from build123d import *

# Parameters (mm, degrees)
BOSS_EXTRUDE1_DEPTH          = 2
SKETCH2_W                    = 2
SKETCH2_H                    = 25
CUT_EXTRUDE_THIN1_DEPTH      = 1
CUT_EXTRUDE_THIN1_DEPTH_BACK = 3


with BuildPart() as part:
    # Sketch1 → Boss-Extrude1 (new body)
    with BuildSketch(Plane(origin=(0, 0, 0), x_dir=(1, 0, 0), z_dir=(0, 1, 0))):
        Polygon((-20.207259422, -35), (20.207259422, -35), (40.414518843, 0), (20.207259422, 35), (-20.207259422, 35), (-40.414518843, 0), align=None)
    extrude(amount=BOSS_EXTRUDE1_DEPTH)

    # Sketch2 → Cut-Extrude-Thin1 (cut, two sides)
    with BuildSketch(Plane(origin=(0, 2, 0), x_dir=(1, 0, 0), z_dir=(0, 1, 0))) as cut_extrude_thin1_sk:
        with Locations((0, 12.5)):
            Rectangle(SKETCH2_W, SKETCH2_H)
    extrude(amount=CUT_EXTRUDE_THIN1_DEPTH, mode=Mode.SUBTRACT)
    extrude(cut_extrude_thin1_sk.sketch, amount=-CUT_EXTRUDE_THIN1_DEPTH_BACK, mode=Mode.SUBTRACT)


solid = part.part
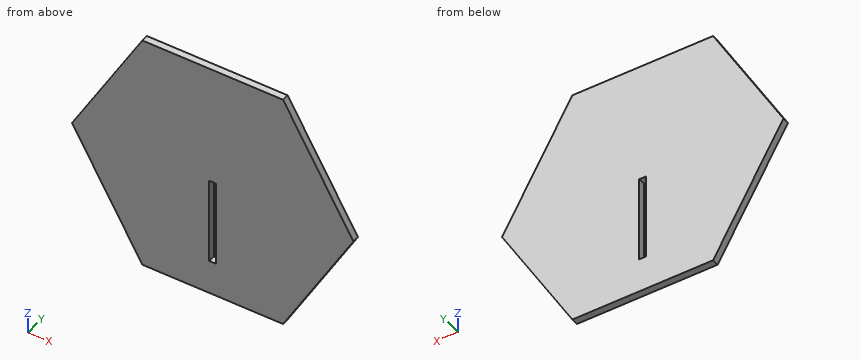
Could you check a few things on this model? Use its own coordinates, in mm. Round coordinates to 2 decimals unless told otherwise and drop trailing zeros. Order: outer loops, then holes, each group sorted by start corner. A loop starts at its lowest first (then second) coordinate and runs counter-clockwise, first axis right, second up.
(1) Imagine slicing it at C-C (x = -24). Write out the boundary of the cut face in (y, z).
Response values:
outline: (0, -28.43) - (2, -28.43) - (2, 28.43) - (0, 28.43) - close
(2) Imagine slicing it at D-D (z = 21.5). Write out the boundary of the cut face in (x, y).
Response values:
outline: (-28, 0) - (28, 0) - (28, 2) - (-28, 2) - close
(3) Please list where these lines run through material, in increasing order: line 1 along X through (y, z) = (1.65, -19); line 2 along X through (y, z) = (0.6, -12.5); line 3 along X through (y, z) = (1.05, 3).
Response values:
line 1: x = -29.44 to -1, 1 to 29.44
line 2: x = -33.2 to -1, 1 to 33.2
line 3: x = -38.68 to 38.68
(4) Imagine slicing it at A-A (y = 1.5). Write out the boundary of the cut face in (x, z).
Response values:
outline: (-40.41, 0) - (-20.21, -35) - (20.21, -35) - (40.41, 0) - (20.21, 35) - (-20.21, 35) - close; hole (-1, -25) - (1, -25) - (1, 0) - (-1, 0) - close
(5) Imagine slicing it at B-B (z = -4). Write out the boundary of the cut face in (x, y).
Response values:
outline: (-38.11, 0) - (-1, 0) - (-1, 2) - (-38.11, 2) - close; (1, 0) - (38.11, 0) - (38.11, 2) - (1, 2) - close
(6) I'm going to push flat-ended pins straight in: pin 1 (1 mm diameter, centred on y = 1.5, z = 26, fed in from -X); pin 2 (0.6 mm diameter, centred on y = 1.5, z = -11.5, fed in from +X). Where does each tip first touch, or does it pass through?
Response values:
pin 1: stops at x = -25.69
pin 2: stops at x = 33.95
